```python
from build123d import *

# Parameters (mm, degrees)
CROQUIS1_W              = 190
CROQUIS1_H              = 190
CROQUIS1_R              = 1.5
CROQUIS1_R_2            = 2.6
CROQUIS1_W_2            = 45.75
CROQUIS1_H_2            = 150
CROQUIS1_W_3            = 40.5
CROQUIS1_W_4            = 5
CROQUIS1_H_3            = 7
CROQUIS1_W_5            = 7
CROQUIS1_H_4            = 5
SALIENTE_EXTRUIR1_DEPTH = 2
CROQUIS2_W              = 190
CROQUIS2_H              = 190
CROQUIS2_W_2            = 180
CROQUIS2_H_2            = 180
CORTAR_EXTRUIR1_DEPTH   = 74


with BuildPart() as part:
    # Croquis1 → Saliente-Extruir1 (new body)
    with BuildSketch(Plane(origin=(0, 0, 0), x_dir=(1, 0, 0), z_dir=(0, 1, 0))):
        with Locations((85, 85)):
            Rectangle(CROQUIS1_W, CROQUIS1_H)
        with Locations(Location((60.25, 109.75, 0), (0, 0, 270))):
            Circle(CROQUIS1_R, mode=Mode.SUBTRACT)
        with Locations(Location((60.25, 60.25, 0), (0, 0, 270))):
            Circle(CROQUIS1_R, mode=Mode.SUBTRACT)
        with Locations(Location((0, 170, 0), (0, 0, 270))):
            Circle(CROQUIS1_R_2, mode=Mode.SUBTRACT)
        with Locations(Location((0, 0, 0), (0, 0, 270))):
            Circle(CROQUIS1_R_2, mode=Mode.SUBTRACT)
        with Locations(Location((109.75, 109.75, 0), (0, 0, 90))):
            Circle(CROQUIS1_R, mode=Mode.SUBTRACT)
        with Locations(Location((109.75, 60.25, 0), (0, 0, 90))):
            Circle(CROQUIS1_R, mode=Mode.SUBTRACT)
        with Locations(Location((170, 0, 0), (0, 0, 90))):
            Circle(CROQUIS1_R_2, mode=Mode.SUBTRACT)
        with Locations(Location((170, 170, 0), (0, 0, 90))):
            Circle(CROQUIS1_R_2, mode=Mode.SUBTRACT)
        with Locations((32.875, 85)):
            Rectangle(CROQUIS1_W_2, CROQUIS1_H_2, mode=Mode.SUBTRACT)
        with Locations((137.125, 85)):
            Rectangle(CROQUIS1_W_2, CROQUIS1_H_2, mode=Mode.SUBTRACT)
        with Locations((85, 85)):
            Rectangle(CROQUIS1_W_3, CROQUIS1_H_2, mode=Mode.SUBTRACT)
        with Locations((170, 85)):
            Rectangle(CROQUIS1_W_4, CROQUIS1_H_3, mode=Mode.SUBTRACT)
        with Locations((85, 170)):
            Rectangle(CROQUIS1_W_5, CROQUIS1_H_4, mode=Mode.SUBTRACT)
    extrude(amount=SALIENTE_EXTRUIR1_DEPTH)

    # Croquis2 → Cortar-Extruir1 (cut)
    with BuildSketch(Plane(origin=(0, 2, 0), x_dir=(1, 0, 0), z_dir=(0, 1, 0))):
        with Locations((85, 85)):
            Rectangle(CROQUIS2_W, CROQUIS2_H)
        with Locations((85, 85)):
            Rectangle(CROQUIS2_W_2, CROQUIS2_H_2, mode=Mode.SUBTRACT)
    extrude(amount=-CORTAR_EXTRUIR1_DEPTH, mode=Mode.SUBTRACT)


solid = part.part
```
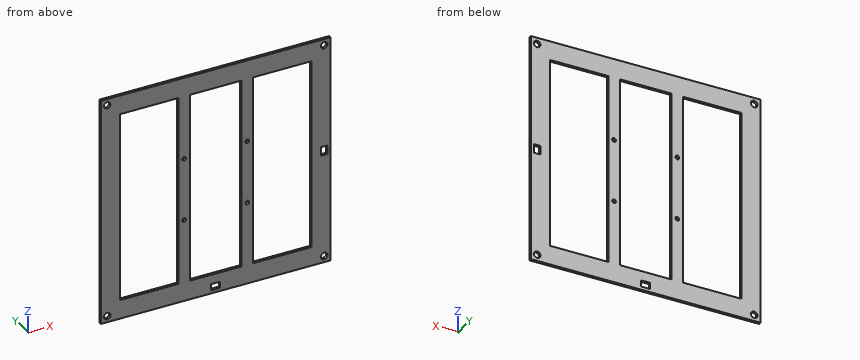
Geometry: final body of the model. Coordinates: model frame, mm. Round coordinates to 2 decimals unless told otherwise and drop trailing zeros. Order: outer loops, then holes, each group sorted by start corner. A loop starts at its lowest first (then second) coordinate and runs counter-clockwise, first axis right, second up. Notation, with made-up numbers: M -18,59 L 0,59 A18 ccw 0,90 Z; hole C 28.25,-3 d5. An arc over 180 degrees is marked long. One line per item, written item: value.
(1) Cut plane C-C (y = 1.7). Give the number of separate pieces and of enclosed holes in the cut face, and give its area (3 significant figures).
Result sheet:
separate pieces: 1
enclosed holes: 13
area: 12,400 mm2
(2) Cut plane A-A (z = -70). Return the cut outline in (x, y).
Result sheet:
outline: M -5,0 L 10,0 L 10,2 L -5,2 Z; M 55.75,0 L 64.75,0 L 64.75,2 L 55.75,2 Z; M 105.25,0 L 114.25,0 L 114.25,2 L 105.25,2 Z; M 160,0 L 175,0 L 175,2 L 160,2 Z
(3) Pin query (flat end, axial travel): P1, Ø2.5, axis at x = 60.25, z = -109.75, coming from the +Y side; P2, Ø8.5, axis at x = 170, z = 0, coming from the +Y side. Return the tip coordinate at first contact, or that it passes through.
Result sheet:
P1: through
P2: y = 2
(4) Cut plane B-B (x = 95). Return the cut outline in (y, z).
Result sheet:
outline: M 0,-175 L 2,-175 L 2,-160 L 0,-160 Z; M 0,-10 L 2,-10 L 2,5 L 0,5 Z
(5) Cut plane D-D (z = -170). Return the cut outline in (x, y), and give its area (3 significant figures).
Result sheet:
outline: M -5,0 L -2.6,0 L -2.6,2 L -5,2 Z; M 2.6,0 L 81.5,0 L 81.5,2 L 2.6,2 Z; M 88.5,0 L 167.4,0 L 167.4,2 L 88.5,2 Z; M 172.6,0 L 175,0 L 175,2 L 172.6,2 Z
area: 325 mm2
(6) Line query: probe 1 along X at (y, z) = (1.25, -31); probe 2 along X at (y, z) = (1.2, 0); probe 3 along X at (y, z) = (0.5, -83.5). Output: solid intervals per line, ascending. Write a range as [from, to].
Result sheet:
probe 1: [-5, 10], [55.75, 64.75], [105.25, 114.25], [160, 175]
probe 2: [-5, -2.6], [2.6, 167.4], [172.6, 175]
probe 3: [-5, 10], [55.75, 64.75], [105.25, 114.25], [160, 167.5], [172.5, 175]
